Model file for the job. Use its own axes, mm. A direction names the side the tool comes from. Give positions to 0.01 mm unless a question says otherwise; leave off trailing zeros. Write each loop counter-clockwise with the first axis right and the second up, starting at its lowest first coordinate (ties: lowest second). Pieces come first, ordered by that corner, then holes.
```python
from build123d import *

# Parameters (mm, degrees)
SALIENTE_EXTRUIR1_DEPTH    = 10
CROQUIS2_OUTSIDE_W         = 34.364
CROQUIS2_OUTSIDE_H         = 70.364
CROQUIS2_OUTSIDE_W_2       = 8
CROQUIS2_OUTSIDE_H_2       = 8
CORTAR_EXTRUIR2_DEPTH      = 10
CROQUIS3_R                 = 2
CORTAR_EXTRUIR3_DEPTH      = 33.445689749
CORTAR_EXTRUIR4_DEPTH      = 31.9309357
CORTAR_EXTRUIR4_DEPTH_BACK = 31.9309357
CROQUIS6_R                 = 50
REDONDEO1_R                = 1
REDONDEO3_R                = 4


with BuildPart() as part:
    # Croquis1 → Saliente-Extruir1 (new, symmetric)
    with BuildSketch(Plane(origin=(0, 0, 0), x_dir=(0, 0, -1), z_dir=(1, 0, 0))):
        with BuildLine():
            Line((-28, 10), (28, 10))
            Line((28, 10), (28, 3.096227789))
            ThreePointArc((28, 3.096227789), (24.352048797, -4.627209016), (16.069704783, -6.715701704))
            ThreePointArc((16.069704783, -6.715701704), (0, -5.150015015), (-16.069704783, -6.715701704))
            ThreePointArc((-16.069704783, -6.715701704), (-24.352048797, -4.627209016), (-28, 3.096227789))
            Line((-28, 3.096227789), (-28, 10))
        make_face()
    extrude(amount=SALIENTE_EXTRUIR1_DEPTH, both=True)

    # Croquis2 outside → Cortar-Extruir2 (cut)
    with BuildSketch(Plane(origin=(0, 10, 0), x_dir=(1, 0, 0), z_dir=(0, 1, 0))):
        Rectangle(CROQUIS2_OUTSIDE_W, CROQUIS2_OUTSIDE_H)
        Rectangle(CROQUIS2_OUTSIDE_W_2, CROQUIS2_OUTSIDE_H_2, mode=Mode.SUBTRACT)
    extrude(amount=-CORTAR_EXTRUIR2_DEPTH, mode=Mode.SUBTRACT)

    # Croquis3 → Cortar-Extruir3 (cut, through all)
    with BuildSketch(Plane.ZY.offset(4)):
        with Locations((0, 5)):
            Circle(CROQUIS3_R)
    extrude(amount=-CORTAR_EXTRUIR3_DEPTH, mode=Mode.SUBTRACT)

    # Croquis6 → Cortar-Extruir4 (cut, two sides: drawn at the far end of the back side and taken through both)
    with BuildSketch(Plane.XY.offset(-CORTAR_EXTRUIR4_DEPTH_BACK)):
        with Locations((0, -55.893567066)):
            Circle(CROQUIS6_R)
    extrude(amount=CORTAR_EXTRUIR4_DEPTH + CORTAR_EXTRUIR4_DEPTH_BACK, mode=Mode.SUBTRACT)

    # Redondeo1
    redondeo1_edges = [part.edges().sort_by_distance(p)[0] for p in [
        (-10, 0, 0),
        (0, 0, -27.508594716),
        (0, 0, 27.508594716),
        (10, 0, 0),
        (0, 0, -4),
        (-4, 0, 0),
        (0, 0, 4),
        (4, 0, 0),
    ]]
    fillet(redondeo1_edges, radius=REDONDEO1_R)

    # Redondeo3
    redondeo3_edges = [part.edges().sort_by_distance(p)[0] for p in [
        (0, 10, -4),
        (0, 10, 4),
    ]]
    fillet(redondeo3_edges, radius=REDONDEO3_R - 0.0001)  # a hair under: the kernel refuses the full size


solid = part.part
```
1. Which spindle directions (+Z, -Z, +X, -X, +Y, -Y) get a long thin tool onto all of the face, cutting with end or side? Do faces 4 (the flat face through (4, 7, -2)), 5 (the flat face through (0, 4, 4)), 6 (the cylindrical face through (-9.728, -6.796, -16.535)). Say none if no direction does.
Calculated:
face 4: +Z, -Z, +X, +Y
face 5: +Z, +X, -X, +Y
face 6: +X, -X, -Y
2. Pin check, flat tips, straight feed: P1, Ø5, axis at y = 5, z = 0, coming from the -X side; P2, Ø1.5, axis at x = 2.5, z = 5, coming from the -Y side; P3, Ø5.5, axis at x = 2, y = 3.5, coming from the -Z side. Stop position of each tip, or through.
Calculated:
P1: stops at x = -4
P2: stops at y = -5.35
P3: stops at z = -4.03
3. Slice it at C-C, the plane z = -12. Write the cut outline in (x, y), and give its area (3 significant figures).
Calculated:
outline: (-10, -6.02) - (-3.55, -6.02) arc R50 cw to (3.55, -6.02) - (10, -6.02) - (10, -1) arc R1 ccw to (9, 0) - (-9, 0) arc R1 ccw to (-10, -1) - close
area: 119 mm2
4. Probe probe 1 along Y at (x, z) = (1.5, 0); probe 2 along Z at (x, y) = (-1.75, 5.5); probe 3 along Y at (x, z) = (-9, -19). List the from-to ranges inside material, lowest first.
Calculated:
probe 1: y = -5.15 to 3, 7 to 10
probe 2: z = -4 to -1.94, 1.94 to 4
probe 3: y = -6.71 to 0
5. Pull direction Z, two halves, no side cores. Call faces 1 (the cylindrical face through (-9.692, -6.795, 16.526)), 2 (the cylindrical face through (0.14, -3.864, -25.18)), 3 (the cylindrical face through (-4.285, 0.301, -0.07)): +Z half, -Z half, draft (parallel to the pull), parting line (faces both ways), or undercut.
Calculated:
face 1: undercut
face 2: -Z half
face 3: draft
6. Slice it at A-A, the plane y = 5. Write the cut outline in (x, z).
Calculated:
outline: (-4, -4) - (4, -4) - (4, -2) - (-4, -2) - close; (-4, 2) - (4, 2) - (4, 4) - (-4, 4) - close
